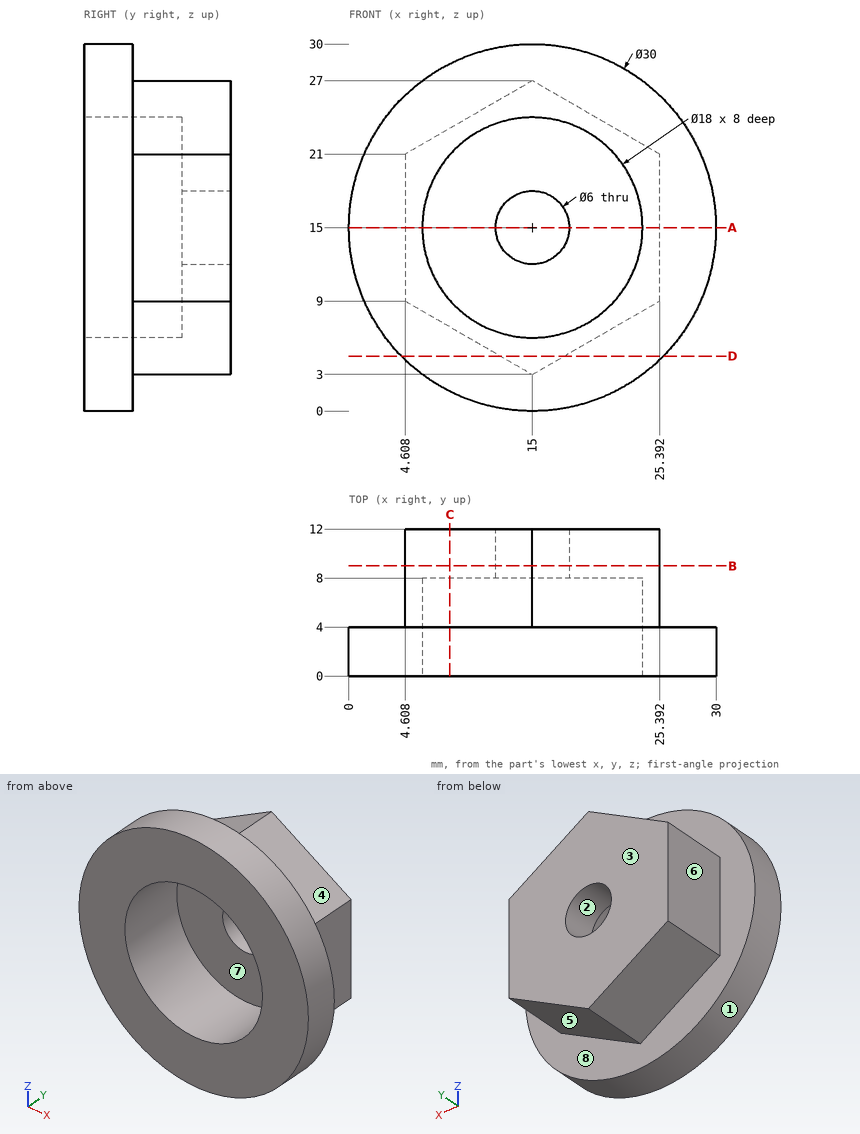
Input: dimensioned drawing with shaded views. Units: mm. Origin: part minimum x, y, z. A direction names the side the tool comes from. Round coordinates to 2 decimals unless told otherwise and drop trailing zeros. Order: outer loops, then holes, each group sorted by start corner. A loop starts at its lowest first (then second) coordinate and runs counter-clockwise, first axis right, second up. Notation, with made-up numbers: (-17, -24.75) - (-4, -24.75) arc R19 cw to (-4, -3.75) - close; hole circle Ø11 at (-1.75, 35.25). An arc over 180 degrees is marked (long way). Use CSV: the item, a comma, the result in double quotes. Start each with the question number.
Q1. Mould query, pull axis Z, two halves, no side actions, for the marked faces 1, 2 and 3. Classes: +Z half, -Z half, draft (parallel to the pull), parting line (faces both ways), or undercut.
Q2. Material intervals for line 1 along Z through (x, y) = (15, 2); line 2 along X through (y, z) = (10.7, 15); line 3 along Y through (x, z) = (4, 20.75), sorted ascending. Write a range as from..to.
Q3. First-contact query: pin 1 (5 mm diameter, centred on y = 10.5, z = 25.5, fed in from +X); pin 2 (2.5 mm diameter, centred on y = 7.5, z = 15.5, fed in from -X); pin 3 (2 mm diameter, centred on y = 5.5, z = 5.5, fed in from +X); pin 4 (1 mm diameter, centred on x = 8, z = 10, fed in from -Y). Flat tips, straight axial feed; report the tip coordinate or a pass-through.
Q4. Section query B-B (y = 9). Return loops of the section in (x, z).
Q5. Section query D-D (z = 4.5). Return loops of the section in (x, y), and give its area (3 significant figures).
Q6. Access query for the marked faces 4, 5, 6, 7 and 8. Directions: +Z, -Z, +X, -X, +Y, -Y. A direction counts if a zero-diameter tool reaches every point of the face in a straight line with its end or side. Return the directions, or none.
Q7. Section query C-C (x = 8.25). Return loops of the section in (y, z) (1 decimal).
Q8. Section query A-A (z = 15). Return loops of the section in (x, y).
Result set:
1,face 1,"parting line"
1,face 2,"undercut"
1,face 3,"draft"
2,line 1,"z = 0..6, 24..30"
2,line 2,"x = 4.61..12, 18..25.39"
2,line 3,"y = 0..4"
3,pin 1,"stops at x = 21.93"
3,pin 2,"stops at x = 4.61"
3,pin 3,"stops at x = 21.06"
3,pin 4,"stops at y = 0"
4,outline,"(4.61, 9) - (15, 3) - (25.39, 9) - (25.39, 21) - (15, 27) - (4.61, 21) - close; hole circle Ø6 at (15, 15)"
5,outline,"(4.29, 0) - (25.71, 0) - (25.71, 4) - (17.6, 4) - (17.6, 12) - (12.4, 12) - (12.4, 4) - (4.29, 4) - close"
5,area,"127 mm2"
6,face 4,"+Z, +X, +Y"
6,face 5,"-Z, +X, +Y"
6,face 6,"+Z, -Z, -X, +Y"
6,face 7,"-Y"
6,face 8,"+Y"
7,outline,"(0, 1.6) - (4, 1.6) - (4, 6.9) - (12, 6.9) - (12, 23.1) - (4, 23.1) - (4, 28.4) - (0, 28.4) - (0, 21) - (8, 21) - (8, 9) - (0, 9) - close"
8,outline,"(0, 0) - (6, 0) - (6, 8) - (12, 8) - (12, 12) - (4.61, 12) - (4.61, 4) - (0, 4) - close; (18, 8) - (24, 8) - (24, 0) - (30, 0) - (30, 4) - (25.39, 4) - (25.39, 12) - (18, 12) - close"
